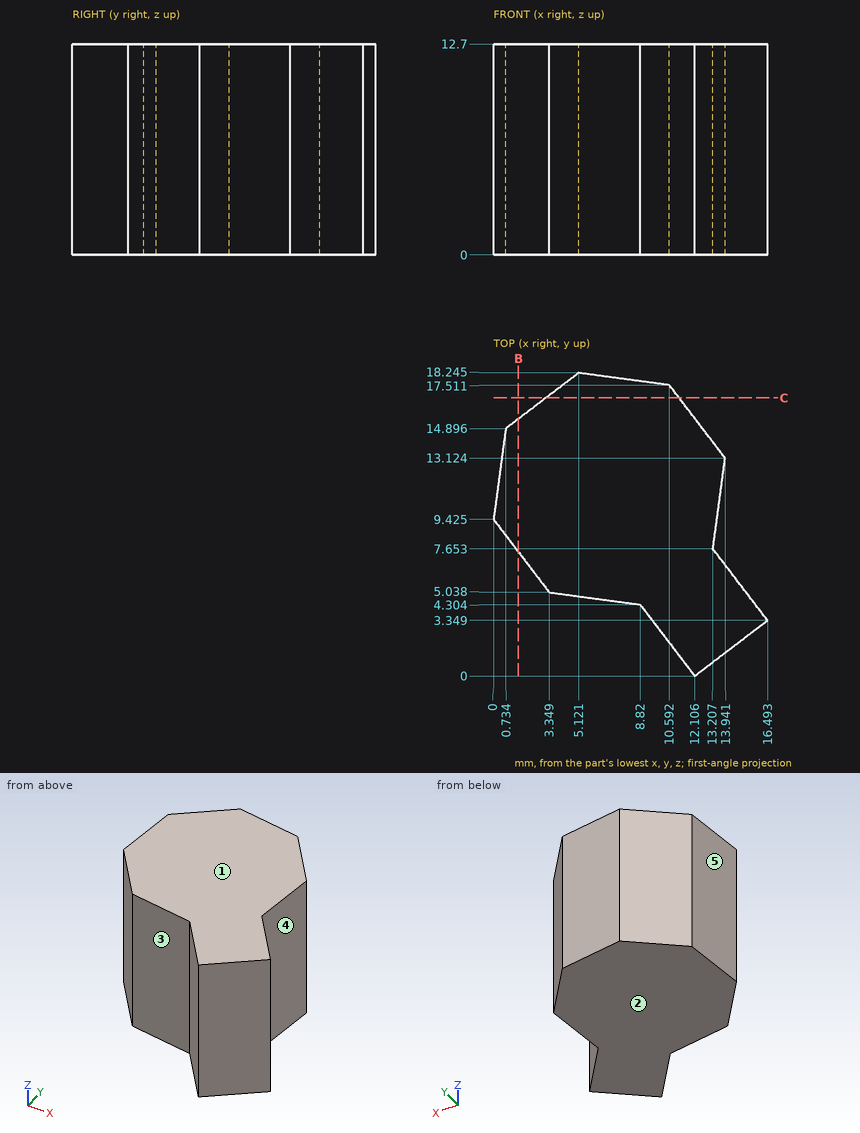
The figure shows three views and two pictorial views of one solid part (mm, origin at its lowest corner). Answer the questions. A direction names the side the tool comes from. Give positions to 0.01 mm unless a question says otherwise; leave off trailing zeros. Loops run counter-clockwise (first coordinate to the right, second up) from the corner with the lowest first, then second, coordinate; pieces in that order, holes last. Notation, with made-up numbers: (40.25, 81) -> (94.25, 81) arc R36 ccw to (94.25, 119) -> close; hole circle Ø7 at (-15, -12.5). An arc over 180 degrees is marked (long way). Put each result on its own line as item: value. Start each with the question number.
Item 1: The mould has two halves that part along Z. Classify the marked faces 1, 2 and 3: released by +Z, released by -Z, zero draft, split by the parting line, or undercut.
Item 2: Find the intervals of material crossed by L1, parallel to X at y = 13.5, z = 8.75 (1 decimal); L2, parallel to X at y = 3.5, z = 5 (1 decimal); L3, parallel to Y at x = 1.75, z = 1 (1 decimal), in increasing order. Write a range as [from, to].
Item 3: The part is cut by section B-B (x = 1.5). Give the vertices of the cut face in (y, z).
Item 4: Which of the six approach directions +Z, -Z, +X, -X, +Y, -Y give full straight-line access (tool end or side, diameter ignored) to the marked faces 4 and 5?
Item 5: The part is cut by section C-C (y = 16.75). Give the vertices of the cut face in (x, z).
Item 6: Each of these flat-tipped pins is pushed along its axis until it touches: P1, Ø6, axis at x = 12, z = 9.5, coming from the +Y side (1 decimal); P2, Ø4, axis at x = 8, z = 3.5, coming from the -Y side; P3, Ø3, axis at x = 11.5, z = 10.5, coming from the +Y side. Where does it stop, or does it pass through?
Answers below:
1. face 1: released by +Z
1. face 2: released by -Z
1. face 3: zero draft
2. L1: [0.5, 13.7]
2. L2: [9.4, 16.4]
2. L3: [7.1, 15.7]
3. outline: (7.46, 0) -> (15.48, 0) -> (15.48, 12.7) -> (7.46, 12.7) -> close
4. face 4: +Z, -Z, +X
4. face 5: +Z, -Z, -X, +Y
5. outline: (3.16, 0) -> (11.17, 0) -> (11.17, 12.7) -> (3.16, 12.7) -> close
6. P1: y = 17.7
6. P2: y = 2.76
6. P3: y = 17.59
